Geometry: final body of the model. Coordinates: model frame, mm. A direction names the side the tool comes from. Give positions to 0.01 mm unless a question says otherwise; leave off trailing zeros. Write each loop counter-clockwise with the first axis right and the second up, starting at its lowest first coordinate (ties: lowest second). Pieces come first, ordered by that corner, then holes. Notation, with made-up numbers: (76, 10) -> (81, 10) arc R8 cw to (81, 25) -> close; hole circle Ø11 at (73.5, -19.5). An arc over 180 degrees is marked (long way). Answer as a JSON object with one key per item and string values.
from build123d import *

# Parameters (mm, degrees)
SKETCH_2_R               = 5
SKETCH_2_R_2             = 1.999999992
EXTRUDE_1_DEPTH          = 9
CUT_EXTRUDE_1_DEPTH      = 170.859032113
CUT_EXTRUDE_1_DEPTH_BACK = 170.859032113
SKETCH_4_R               = 5
CUT_EXTRUDE_2_DEPTH      = 170.478188001


with BuildPart() as part:
    # 草图2 → 凸台-拉伸1 (new body)
    with BuildSketch(Plane.XY):
        with BuildLine():
            Line((147.519937563, 5.502226824), (12.479900949, 5.500188388))
            ThreePointArc((12.479900949, 5.500188388), (8.429429601, 6.057352235), (4.679877945, 7.687570645))
            ThreePointArc((4.679877945, 7.687570645), (-4.365546387, 7.87032431), (-8.999445953, 0.099862608))
            Line((-8.999445953, 0.099862608), (-8.999442934, -0.100134306))
            ThreePointArc((-8.999442934, -0.100134306), (-4.365308776, -7.870456104), (4.680110035, -7.687429353))
            ThreePointArc((4.680110035, -7.687429353), (8.429612472, -6.057097743), (12.480066997, -5.499811611))
            Line((12.480066997, -5.499811611), (147.520099033, -5.497773175))
            ThreePointArc((147.520099033, -5.497773175), (151.570570386, -6.054937034), (155.320122044, -7.68515546))
            ThreePointArc((155.320122044, -7.68515546), (164.365546377, -7.867909125), (168.999445942, -0.097447423))
            Line((168.999445942, -0.097447423), (168.999442923, 0.102549491))
            ThreePointArc((168.999442923, 0.102549491), (164.365308765, 7.87287129), (155.319889955, 7.689844539))
            ThreePointArc((155.319889955, 7.689844539), (151.570389715, 6.05951356), (147.519937563, 5.502226824))
        make_face()
        Circle(SKETCH_2_R, mode=Mode.SUBTRACT)
        with Locations((159.999999989, 0.002415185)):
            Circle(SKETCH_2_R_2, mode=Mode.SUBTRACT)
    extrude(amount=EXTRUDE_1_DEPTH)

    # 草图3 → 切除-拉伸1 (cut, two sides: drawn at the far end of the back side and taken through both)
    with BuildSketch(Plane(origin=(-8.3023e-05, 5.500000002, 0), x_dir=(0.9999999998860698, 1.509504600630928e-05, 0), z_dir=(-1.509504600630928e-05, 0.9999999998860698, 0)).offset(-CUT_EXTRUDE_1_DEPTH_BACK)):
        Polygon((21.000555556, -4), (26.000555556, -9), (-8.999444444, -9), (-8.999444444, -4), align=None)
        Polygon((29.000555556, -5), (24.000555556, 0), (168.999444452, 0), (168.999444452, -5), align=None)
    extrude(amount=CUT_EXTRUDE_1_DEPTH + CUT_EXTRUDE_1_DEPTH_BACK, mode=Mode.SUBTRACT)

    # 草图4 → 切除-拉伸2 (cut, through all)
    with BuildSketch(Plane.XY.offset(9)):
        with Locations((159.999999989, 0.002415185)):
            Circle(SKETCH_4_R)
    extrude(amount=-CUT_EXTRUDE_2_DEPTH, mode=Mode.SUBTRACT)


solid = part.part
Q1. First-contact query: P1, Ø8, axis at x = 41.5, y = 3.5, coming from the -Z side; P2, Ø1.5, axis at y = -6.5, z = 4.5, coming from the -X side; P3, Ø2, axis at x = 26.5, y = 2, coming from the -Z side. Flat tips, straight axial feed; report the tip coordinate or a pass-through.
Values:
{"P1": "z = 5", "P2": "x = -6.76", "P3": "z = 1.5"}
Q2. Cut plane B-B (y = -1.75). Return the cut outline in (x, z).
Values:
{"outline": "(-8.83, 0) -> (-4.68, 0) -> (-4.68, 4) -> (-8.83, 4) -> close; (4.68, 0) -> (24, 0) -> (29, 5) -> (155.32, 5) -> (155.32, 9) -> (26, 9) -> (21, 4) -> (4.68, 4) -> close; (164.68, 5) -> (168.83, 5) -> (168.83, 9) -> (164.68, 9) -> close"}
Q3. Set-up query: faces 1 (the flat face through (6, 0, 4)), 2 (the flat face through (96, 0, 9)), 3 (the flat face through (100, 0, 5)). Return all of +Z, -Z, +X, -X, +Y, -Y with unobstructed straight access to the full face (end or side cutting, diameter ignored); none if empty.
Values:
{"face 1": "+Z, -X, +Y, -Y", "face 2": "+Z, +X, -X, +Y, -Y", "face 3": "-Z, +X, +Y, -Y"}
Q4. Cut plane A-A (x = 0). Return the cut outline in (y, z), and give its area (3 significant figures).
Values:
{"outline": "(-9, 0) -> (-5, 0) -> (-5, 4) -> (-9, 4) -> close; (5, 0) -> (9, 0) -> (9, 4) -> (5, 4) -> close", "area": "32.0 mm²"}
Q5. Cut plane C-C (x = 66). Return the cut outline in (y, z), and give its area (3 significant figures).
Values:
{"outline": "(-5.5, 5) -> (5.5, 5) -> (5.5, 9) -> (-5.5, 9) -> close", "area": "44.0 mm²"}
Q6. Material intervals for L1, parallel to Y at x = 0, z = 1.55; L2, parallel to Z at x = 89.5, y = 1; L3, parallel to X at y = 0.25, z = 2, sorted ascending. Write a range as from..to.
Values:
{"L1": "-9..-5, 5..9", "L2": "5..9", "L3": "-9..-4.99, 4.99..26"}
Q7. Mould query, pull axis X, two halves, no side actions, for faces 4 (the cylindrical face through (151.626, 6.075, 6.972)), 5 (the cylindrical face through (164.77, 1.5, 7.03)), 6 (the cylindrical face through (-1.08, -4.88, 1.97)), 7 (the flat face through (7, 0, 0)). Classes: pulls with the +X half, pulls with the -X half, needs draft (parallel to the pull), parting line crosses it, or undercut.
Values:
{"face 4": "pulls with the -X half", "face 5": "undercut", "face 6": "undercut", "face 7": "needs draft"}
